Here's how the part is built. I have some questions about the finished solid (model axes, mm). A direction names the side the tool comes from. Round coordinates to 2 decimals unless told otherwise and drop trailing zeros. Order: outer loops, then holes, each group sorted by start corner. A loop starts at its lowest first (then second) coordinate and runs counter-clockwise, first axis right, second up. Notation, with made-up numbers: (7.5, 10.5) -> (19.5, 10.5) arc R29 ccw to (19.5, 40.5) -> close; hole circle Ø5 at (-18, 11.25). An arc over 180 degrees is marked (long way). Answer in a Markdown table with one row per item.
```python
from build123d import *

# Parameters (mm, degrees)
SKETCH1_R           = 1.75
SKETCH1_R_2         = 3
BOSS_EXTRUDE2_DEPTH = 6


with BuildPart() as part:
    # Sketch1 → Boss-Extrude2 (new body)
    with BuildSketch(Plane.XY):
        Polygon((72, 72), (32, 72), (32, 78), (-38, 78), (-38, 72), (-72, 72), (-72, 56.2), (-67.772810154, 56.2), (-67.772810154, 57.6), (-64.957983727, 57.6), (-64.957983727, 56.2), (-60, 56.2), (-60, 53), (-64.957983727, 53), (-64.957983727, 51.568504207), (-67.772810154, 51.568504207), (-67.772810154, 53), (-72, 53), (-72, 38), (-78, 38), (-78, -32), (-72, -32), (-72, -50.4), (-67.78187279, -50.4), (-67.78187279, -49), (-64.967046362, -49), (-64.967046362, -50.4), (-60, -50.4), (-60, -53.6), (-64.967046362, -53.6), (-64.967046362, -55), (-67.78187279, -55), (-67.78187279, -53.6), (-72, -53.6), (-72, -72), (-38, -72), (-38, -66), (-4.6, -66), (-4.6, -60.77149924), (-6, -60.77149924), (-6, -57.77149924), (-4.6, -57.77149924), (-4.6, -54), (-1.4, -54), (-1.4, -57.77149924), (0, -57.77149924), (0, -60.77149924), (-1.4, -60.77149924), (-1.4, -66), (32, -66), (32, -72), (72, -72), (72, -32), (66, -32), (66, 38), (72, 38), align=None)
        with Locations((69, -52)):
            Circle(SKETCH1_R, mode=Mode.SUBTRACT)
        Circle(SKETCH1_R_2, mode=Mode.SUBTRACT)
        with Locations((69, 55)):
            Circle(SKETCH1_R, mode=Mode.SUBTRACT)
        with Locations((0, 75)):
            Circle(SKETCH1_R, mode=Mode.SUBTRACT)
    extrude(amount=BOSS_EXTRUDE2_DEPTH)


solid = part.part
```
1. For faces 4 (the face through (69, -32, 3)), 5 (the face through (-4.6, -63, 3)), 6 (the face through (-70, -53.6, 3)), 7 (the face through (-72, -41, 3)), 8 (the face through (-55, 72, 3)), which set-ups out of +Z, -Z, +X, -X, +Y, -Y let a thin tool reach every point of the face, with its end or its side?
Numbers:
| item | result |
|---|---|
| face 4 | +Z, -Z, +X |
| face 5 | +Z, -Z, -Y |
| face 6 | +Z, -Z, -X |
| face 7 | +Z, -Z, -X, -Y |
| face 8 | +Z, -Z, -X, +Y |
2. Please list where these lines run through material, in increasing order: line 1 along Y through (x, z) = (69, 3.8); line 2 along Y through (x, z) = (-67.5, 3.8); line 3 along X through (y, z) = (75, 2).
Numbers:
| item | result |
|---|---|
| line 1 | y = -72 to -53.75, -50.25 to -32, 38 to 53.25, 56.75 to 72 |
| line 2 | y = -72 to -55, -49 to 51.57, 57.6 to 72 |
| line 3 | x = -38 to -1.75, 1.75 to 32 |
3. Suppose I cut it at C-C on y = 0. Write out the boundary of the cut face in (x, z).
Numbers:
| item | result |
|---|---|
| outline | (-78, 0) -> (-3, 0) -> (-3, 6) -> (-78, 6) -> close; (3, 0) -> (66, 0) -> (66, 6) -> (3, 6) -> close |
4. Suppose I cut it at D-D on y = -35. Write out the boundary of the cut face in (x, z).
Numbers:
| item | result |
|---|---|
| outline | (-72, 0) -> (72, 0) -> (72, 6) -> (-72, 6) -> close |
5. Suppose I cut it at A-A on y = 75. Write out the boundary of the cut face in (x, z), then the cut area to 3 significant figures.
Numbers:
| item | result |
|---|---|
| outline | (-38, 0) -> (-1.75, 0) -> (-1.75, 6) -> (-38, 6) -> close; (1.75, 0) -> (32, 0) -> (32, 6) -> (1.75, 6) -> close |
| area | 399 mm2 |
6. We'd pull the mould along X, two halves only. Please class faces 1 (the face through (-3, 78, 3)), 2 (the face through (-3, -54, 3)), 3 (the face through (72, 55, 3)): released by +X, released by -X, zero draft, split by the parting line, or undercut.
Numbers:
| item | result |
|---|---|
| face 1 | zero draft |
| face 2 | undercut |
| face 3 | released by +X |
7. For pin 1 Ø1.8 at (x, z) = (-76, 2.5) entering from -Y; pin 2 Ø2.5 at (x, z) = (-67, 4.5) entering from +Y; pin 3 Ø1 at (y, z) = (-51.5, 2.5) entering from -X, each with a flat end and sliding along its axis, tell me the tip position at first contact or that it passes through.
Numbers:
| item | result |
|---|---|
| pin 1 | stops at y = -32 |
| pin 2 | stops at y = 72 |
| pin 3 | stops at x = -60 |
8. Suppose I cut it at B-B on z = 3.7. State how many separate pieces and enclosed holes the cut face has, then the cut area to 3 significant figures.
Numbers:
| item | result |
|---|---|
| separate pieces | 1 |
| enclosed holes | 4 |
| area | 20,500 mm2 |
